from build123d import *

# Parameters (mm, degrees)
F1_DEPTH = 50
F0_W     = 3
F0_H     = 90
F0_W_2   = 65
F0_H_2   = 3
F2_DEPTH = 6
F3_DEPTH = 3
F4_R     = 0.99999
F5_R     = 5


# Not quite as in the source:
# - a fillet or chamfer is up to 0.001 mm smaller than in the source, because OpenCascade refuses the exact size


with BuildPart() as f1:
    # F0 (on Front) → F1 (new body)
    with BuildSketch(Plane.XZ):
        Polygon((-67, 6), (-65, 6), (-65, 9), (-66, 9), (-66, 10), (-69, 10), (-69, 9), (-69, 7), (-69, 6), (-68, 6), align=None)
        Polygon((-72, 3), (-68, 3), (-68, 6), (-69, 6), (-69, 7), (-72, 7), align=None)
        Polygon((-75, 0), (-65, 0), (-65, 3), (-68, 3), (-72, 3), (-72, 7), (-72, 10), (-75, 10), align=None)
    extrude(amount=F1_DEPTH)

    # F0 (on Front) → F2 (join)
    with BuildSketch(Plane.XZ):
        with Locations((-73.5, 55)):
            Rectangle(F0_W, F0_H)
        with Locations((-67.5, 55)):
            Rectangle(F0_W, F0_H)
        with Locations((-32.5, 7.5)):
            Rectangle(F0_W_2, F0_H_2)
        with Locations((-32.5, 1.5)):
            Rectangle(F0_W_2, F0_H_2)
    extrude(amount=F2_DEPTH)

    # F0 (on Front) → F3 (join)
    with BuildSketch(Plane.XZ):
        Polygon((-72, 100), (-72, 10), (-72, 7), (-69, 7), (-69, 9), (-69, 10), (-69, 100), align=None)
        Polygon((-65, 3), (0, 3), (0, 6), (-65, 6), (-67, 6), (-68, 6), (-68, 3), align=None)
    extrude(amount=F3_DEPTH)

    # F4 (radius 1 in the source; OpenCascade refuses exactly that, so slightly less here)
    f4_edges = [f1.edges().sort_by_distance(p)[0] for p in [
        (-66, -25, 9),
    ]]
    fillet(f4_edges, radius=F4_R)

    # F5
    f5_edges = [f1.edges().sort_by_distance(p)[0] for p in [
        (-75, -25, 0),
    ]]
    fillet(f5_edges, radius=F5_R)

    # F6: F1 across plane


with BuildPart() as f1_1:
    add(f1.part)
    add(f1.part.mirror(Plane.YZ))


solid = f1_1.part
Geometry: final body of the model. Coordinates: model frame, mm. A direction names the side the tool comes from. Coordinates: 2 decimals unless noted, no trailing zeros. Loops run counter-clockwise (first coordinate to the right, second up) from the corner with the lowest first, then second, coordinate; pieces in that order, holes last. Notation, with made-up numbers: (78, 29.5) - (125, 29.5) arc R24 cw to (125, 58.5) - close; hole circle Ø9 at (73, 63). An arc over 180 degrees is marked (long way). Put each result on its own line as item: value. Start each with the question number.
Q1. Cut plane C-C, the plane x = 61.5. Return loops of the section in (y, z), and give its area (3 significant figures).
Q2. Cut plane A-A, the plane z = 71.5. Return loops of the section in (x, y).
Q3. Line query: line 1 (X direction, y = -42.5, z = 4.5); line 2 (Z direction, x = 17, y = -2). Output: solid intervals per line, ascending.
Q4. Pull-direction query (Z, two-part tool) for faces 1 (the flat face through (70, -2, 100)), 2 (the flat face through (-65, -28, 1)), 3 (the flat face through (68, -26, 4)); classes: released by +Z, released by -Z, zero draft, split by the parting line, or undercut.
Q5. Pin query (flat end, axial travel): pin 1 Ø2.5 at (x, z) = (23, 1.5) entering from -Y; pin 2 Ø23.5 at (x, y) = (-30.5, -26) entering from +Z; pin 3 Ø3.5 at (x, y) = (-67, -33) entering from +Z; pin 4 Ø1.5 at (x, y) = (70.5, -29.5) entering from +Z. Return the tip coordinate at first contact, or that it passes through.
Q6. Set-up query: faces 4 (the flat face through (65, -28, 1)), 5 (the flat face through (74, -6, 56)), 6 (the flat face through (-69, -5.5, 39.9)). Return all of +Z, -Z, +X, -X, +Y, -Y with unobstructed straight access to the full face (end or side cutting, diameter ignored); none if empty.
Filled sheet:
1. outline: (-6, 0) - (0, 0) - (0, 9) - (-6, 9) - (-6, 6) - (-3, 6) - (-3, 3) - (-6, 3) - close
1. area: 45.0 mm²
2. outline: (-75, -6) - (-72, -6) - (-72, -3) - (-69, -3) - (-69, -6) - (-66, -6) - (-66, 0) - (-75, 0) - close; (66, -6) - (69, -6) - (69, -3) - (72, -3) - (72, -6) - (75, -6) - (75, 0) - (66, 0) - close
3. line 1: -74.97 to -68, 68 to 74.97
3. line 2: 0 to 9
4. face 1: released by +Z
4. face 2: zero draft
4. face 3: undercut
5. pin 1: y = -6
5. pin 2: through
5. pin 3: z = 10
5. pin 4: z = 7
6. face 4: +Z, -Z, -Y
6. face 5: +Z, +X, -X, -Y
6. face 6: +Z, -Y
